The listing builds one solid part. Answer for the finished solid, in the listing's coordinates (mm). Face numbers are marked on the shaded views. A direction names the side the tool comes from. Coordinates: 2 decimals unless noted, no trailing zeros. Order: outer loops, then holes, each group sorted by start corner. A loop starts at its lowest first (then second) coordinate and runs counter-clockwise, first axis right, second up. Notation, with made-up numbers: (59.25, -10.75) -> (72.25, -10.75) arc R7 ccw to (72.25, 1.25) -> close; hole circle Ø8 at (59.25, 70). An arc over 180 degrees is marked (long way). Return JSON: item names as keys, results as strings.
```python
from build123d import *

# Parameters (mm, degrees)
F0_W          = 500
F0_H          = 18
F1_DEPTH      = 150
F1_DEPTH_BACK = 150
F2_DEPTH      = 150
F3_DEPTH      = 150
F3_DEPTH_BACK = 150
F4_DEPTH      = 150
F4_DEPTH_BACK = 50
F5_R          = 4
F6_DEPTH      = 100
F7_W          = 5
F7_H          = 12
F8_DEPTH      = 16


with BuildPart() as f1:
    # F0 (on Front) → F1 (new body, two sides)
    with BuildSketch(Plane.XZ) as f1_sk:
        with Locations((101.0303625649, 22.4941878617)):
            Rectangle(F0_W, F0_H)
    extrude(amount=-F1_DEPTH)
    extrude(f1_sk.sketch, amount=F1_DEPTH_BACK)

    # F0 (on Front) → F2 (join)
    with BuildSketch(Plane.XZ):
        Polygon((-148.9696374351, 13.4941878617), (-148.9696374351, 31.4941878617), (-199.4696374351, 81.9941878617), (-199.4696374351, 63.9941878617), (-199.4696374351, 56.538343739), (-156.4254815578, 13.4941878617), align=None)
    extrude(amount=F2_DEPTH)

    # F0 (on Front) → F3 (join, two sides)
    with BuildSketch(Plane.XZ) as f3_sk:
        Polygon((-199.4696374351, 63.9941878617), (-199.4696374351, 81.9941878617), (-306.9254815578, 81.9941878617), (-306.9254815578, 63.9941878617), (-216.3087427616, 63.9941878617), (-206.9254815578, 63.9941878617), align=None)
    extrude(amount=F3_DEPTH)
    extrude(f3_sk.sketch, amount=-F3_DEPTH_BACK)

    # F0 (on Front) → F4 (join, two sides)
    with BuildSketch(Plane.XZ) as f4_sk:
        Polygon((-199.4696374351, 13.4941878617), (-199.4696374351, 56.538343739), (-206.9254815578, 63.9941878617), (-216.3087427616, 63.9941878617), (-216.3087427616, 13.4941878617), align=None)
        Polygon((-199.4696374351, 56.538343739), (-199.4696374351, 63.9941878617), (-206.9254815578, 63.9941878617), align=None)
    extrude(amount=-F4_DEPTH)
    extrude(f4_sk.sketch, amount=F4_DEPTH_BACK)

    # F5 (on face) → F6 (cut)
    with BuildSketch(Plane(origin=(-216.3087427616, 0, 0), x_dir=(0, -1, 0), z_dir=(-1, 0, 0))):
        with Locations((10, 20.4941878617)):
            Circle(F5_R)
    extrude(amount=-F6_DEPTH, mode=Mode.SUBTRACT)

    # F7 (on face) → F8 (cut)
    with BuildSketch(Plane(origin=(0, 0, 13.4941878617), x_dir=(1, 0, 0), z_dir=(0, 0, -1))):
        with Locations((-138.9254815578, 10)):
            Rectangle(F7_W, F7_H)
    extrude(amount=-F8_DEPTH, mode=Mode.SUBTRACT)


solid = f1.part
```
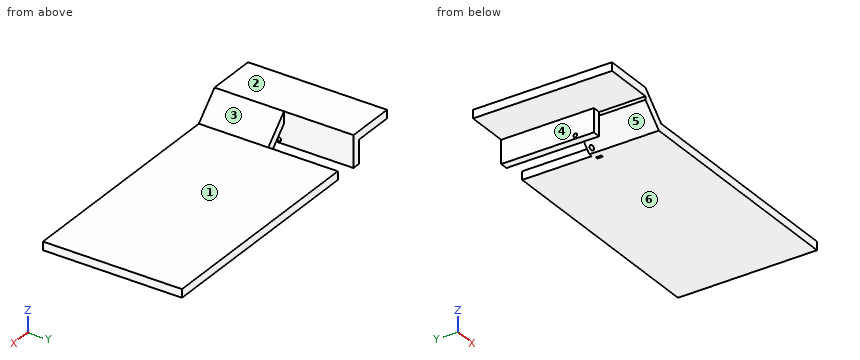
Item 1: Find the intervals of material crossed by probe 1 along Z at (x, y) = (-132, -10); probe 2 along Z at (x, y) = (-207.5, -10); probe 3 along Z at (x, y) = (317, -27), in increasing order.
Answer list:
{"probe 1": "13.49 to 16.49, 24.49 to 31.49", "probe 2": "13.49 to 16.49, 24.49 to 81.99", "probe 3": "13.49 to 31.49"}
Item 2: Determine the mould class of the marked faces 3, 4, 5 and 6 for opening direction X: pulls with the +X half, pulls with the -X half, needs draft (parallel to the pull), parting line crosses it, or undercut.
Answer list:
{"face 3": "pulls with the +X half", "face 4": "pulls with the -X half", "face 5": "undercut", "face 6": "needs draft"}
Item 3: Flat-ended cylindrical pins translate along their axes: pin 1 (9.5 mm diameter, centred on y = -12, z = 22, fed in from -X); pin 2 (6 mm diameter, centred on y = -118, z = 58.5, fed in from -X); pin 3 (25 mm diameter, centred on x = -179, z = 46, fed in from +Y). Find the tip coordinate at first contact, or state that the pin passes through.
Answer list:
{"pin 1": "x = -216.31", "pin 2": "x = -199.47", "pin 3": "y = 0"}
Item 4: The part is cut by section D-D on y = -74.5. Determine the outline of the cut face in (x, z), plus the area to 3 significant figures.
Answer list:
{"outline": "(-306.93, 63.99) -> (-199.47, 63.99) -> (-199.47, 56.54) -> (-156.43, 13.49) -> (351.03, 13.49) -> (351.03, 31.49) -> (-148.97, 31.49) -> (-199.47, 81.99) -> (-306.93, 81.99) -> close", "area": "12,200 mm2"}
Item 5: The part is cut by section B-B on y = -32. Determine the outline of the cut face in (x, z), plus the area to 3 significant figures.
Answer list:
{"outline": "(-306.93, 63.99) -> (-216.31, 63.99) -> (-216.31, 13.49) -> (-199.47, 13.49) -> (-199.47, 56.54) -> (-156.43, 13.49) -> (351.03, 13.49) -> (351.03, 31.49) -> (-148.97, 31.49) -> (-199.47, 81.99) -> (-306.93, 81.99) -> close", "area": "13,000 mm2"}
Item 6: Which of the six approach directions +Z, -Z, +X, -X, +Y, -Y give full straight-line access (tool end or side, diameter ignored) to the marked faces 1 and 2?
Answer list:
{"face 1": "+Z, +X, +Y, -Y", "face 2": "+Z, +X, -X, +Y, -Y"}
Item 7: The part is cut by section C-C on x = 169. Determine the outline of the cut face in (y, z), plus the area to 3 significant figures.
Answer list:
{"outline": "(-150, 13.49) -> (150, 13.49) -> (150, 31.49) -> (-150, 31.49) -> close", "area": "5,400 mm2"}
Item 8: The part is cut by section A-A on y = 30. Determine the outline of the cut face in (x, z), plus the area to 3 significant figures.
Answer list:
{"outline": "(-306.93, 63.99) -> (-216.31, 63.99) -> (-216.31, 13.49) -> (-199.47, 13.49) -> (-199.47, 81.99) -> (-306.93, 81.99) -> close; (-148.97, 13.49) -> (351.03, 13.49) -> (351.03, 31.49) -> (-148.97, 31.49) -> close", "area": "11,800 mm2"}
